from build123d import *

# Parameters (mm, degrees)
SKETCH1_W            = 35
SKETCH1_H            = 35
BOSS_EXTRUDE1_DEPTH  = 3
SKETCH2_R            = 2.5
CUT_EXTRUDE1_DEPTH   = 25.929901725
LPATTERN1_COUNT      = 2
LPATTERN1_PITCH      = 20
LPATTERN1_COUNT_DIR2 = 2
LPATTERN1_PITCH_DIR2 = 20
SKETCH9_R            = 5
SKETCH10_W           = 35
SKETCH10_H           = 35
BOSS_EXTRUDE2_DEPTH  = 3
SKETCH11_R           = 2.5
CUT_EXTRUDE2_DEPTH   = 146.693169663
LPATTERN4_COUNT      = 2
LPATTERN4_PITCH      = 20
LPATTERN4_COUNT_DIR2 = 2
LPATTERN4_PITCH_DIR2 = 20
FILLET1_R            = 3
FILLET2_R            = 3


with BuildPart() as part:
    # Sketch1 → Boss-Extrude1 (new body)
    with BuildSketch(Plane(origin=(0, 0, 0), x_dir=(0, 0, -1), z_dir=(1, 0, 0))):
        Rectangle(SKETCH1_W, SKETCH1_H)
    extrude(amount=BOSS_EXTRUDE1_DEPTH)

    # Sketch2 → Cut-Extrude1 (cut, through all)
    with BuildSketch(Plane(origin=(3, 0, 0), x_dir=(0, 0, -1), z_dir=(1, 0, 0))):
        with Locations((10, 10)):
            Circle(SKETCH2_R)
    cut_extrude1 = extrude(amount=-CUT_EXTRUDE1_DEPTH, mode=Mode.SUBTRACT)

    # LPattern1: Cut-Extrude1 2 × 2
    with Locations(*[(0, -j * LPATTERN1_PITCH_DIR2, i * LPATTERN1_PITCH) for i in range(LPATTERN1_COUNT) for j in range(LPATTERN1_COUNT_DIR2) if (i, j) != (0, 0)]):
        add(cut_extrude1, mode=Mode.SUBTRACT)

    # Sweep1: sweep along a path in Sketch8
    with BuildLine(Plane.XY) as sweep1_path:
        Line((3, 0), (50, 0))
        ThreePointArc((50, 0), (67.677670206, 7.32233044), (75.000001, 25.0000005))
        Line((75.000001, 25.0000005), (75.000001, 90))
        ThreePointArc((75.000001, 90), (67.677670383, 107.677669883), (50.0000005, 115.0000005))
        Line((50.0000005, 115.0000005), (25.0000005, 115.0000005))
    # Sketch9 → Sweep1 (sweep)
    with BuildSketch(Plane(origin=(3, 0, 0), x_dir=(0, 0, -1), z_dir=(1, 0, 0))):
        Circle(SKETCH9_R)
    sweep(path=sweep1_path.line)

    # Sketch10 → Boss-Extrude2 (add)
    with BuildSketch(Plane(origin=(25.000002799, 5e-07, 0), x_dir=(0, 0, 1), z_dir=(-0.9999999999999998, -1.9990267318907433e-08, 0))):
        with Locations((0, 114.9999995)):
            Rectangle(SKETCH10_W, SKETCH10_H)
    extrude(amount=BOSS_EXTRUDE2_DEPTH)

    # Sketch11 → Cut-Extrude2 (cut, through all)
    with BuildSketch(Plane(origin=(22.000002799, 4.4e-07, 0), x_dir=(0, 0, 1), z_dir=(-0.9999999999999998, -1.999026737793079e-08, 0))):
        with Locations(Location((9.998977528, 124.998977028, 0), (0, 0, 270))):
            Circle(SKETCH11_R)
    cut_extrude2 = extrude(amount=-CUT_EXTRUDE2_DEPTH, mode=Mode.SUBTRACT)

    # LPattern4: Cut-Extrude2 2 × 2
    with Locations(*[(0, -j * LPATTERN4_PITCH_DIR2, -i * LPATTERN4_PITCH) for i in range(LPATTERN4_COUNT) for j in range(LPATTERN4_COUNT_DIR2) if (i, j) != (0, 0)]):
        add(cut_extrude2, mode=Mode.SUBTRACT)

    # Fillet1
    fillet1_edges = [part.edges().sort_by_distance(p)[0] for p in [
        (25.0000005, 115.0000005, 5),
    ]]
    fillet(fillet1_edges, radius=FILLET1_R)

    # Fillet2
    fillet2_edges = [part.edges().sort_by_distance(p)[0] for p in [
        (3, 0, 5),
    ]]
    fillet(fillet2_edges, radius=FILLET2_R)


solid = part.part
The listing builds one solid part. Answer for the finished solid, in the listing's coordinates (mm). A direction names the side the tool comes from. Round coordinates to 2 decimals unless told otherwise and drop trailing zeros. Order: outer loops, then holes, each group sorted by start corner. A loop starts at its lowest first (then second) coordinate and runs counter-clockwise, first axis right, second up. Notation, with made-up numbers: (63.5, -13) -> (112.5, -13) arc R7 ccw to (112.5, -6) -> close; hole circle Ø5 at (35, 68.5). An arc over 180 degrees is marked (long way). Put each result on its own line as item: value.
Q1. Section B-B, the plane y = 10 is taken. Count the separate pieces of the cut face and the enclosed holes in it, and give its area (3 significant figures).
Results list:
separate pieces: 4
enclosed holes: 0
area: 175 mm^2
Q2. Each of these flat-tipped pins is pushed along its axis until it touches: P1, Ø0.9, axis at x = 2, z = 2.5, coming from the +Y side; P2, Ø3, axis at y = 125, z = -10, coming from the +X side; P3, Ø6.5, axis at y = 105, z = -10, coming from the +X side; P4, Ø12, axis at y = 81, z = 6.5, coming from the +X side. Where does it stop, or does it pass through?
Results list:
P1: y = 17.5
P2: through
P3: x = 25
P4: x = 79.97
Q3. Section C-C, the plane x = 14.5 is taken. Write down the section's boundary in (y, z).
Results list:
outline: circle Ø10 at (0, 0)
Q4. Consider line 1 along Y through (x, z) = (2.1, 10); line 2 along Y through (x, z) = (33, 0.5); line 3 along Y through (x, z) = (22.5, 5.5). Determine where each line is inside the solid, lowest interval first.
Results list:
line 1: -17.5 to -12.5, -7.5 to 7.5, 12.5 to 17.5
line 2: -4.97 to 4.97, 110.03 to 119.97
line 3: 97.5 to 132.5
Q5. Determine the mould class of faces 6 (the flat face through (0, 0, 0)), 7 (the cylindrical face through (23.479, 107.497, -9.891)), 8 (the flat face through (1, -17.5, 0)) for opening direction Y: pulls with the +Y half, pulls with the -Y half, needs draft (parallel to the pull), parting line crosses it, or undercut.
Results list:
face 6: needs draft
face 7: undercut
face 8: pulls with the -Y half
Q6. Section A-A, the plane y = -10 is taken. Write down the section's boundary in (x, z).
Results list:
outline: (0, -17.5) -> (3, -17.5) -> (3, -12.5) -> (0, -12.5) -> close; (0, -7.5) -> (3, -7.5) -> (3, 7.5) -> (0, 7.5) -> close; (0, 12.5) -> (3, 12.5) -> (3, 17.5) -> (0, 17.5) -> close
Q7. Which of the six approach directions +Z, -Z, +X, -X, +Y, -Y give full straight-line access (tool end or side, diameter ignored) to faces 1 (the flat face through (22, 115, 0)), 2 (the cylindrical face through (1.52, 7.56, 10.54)), 3 (the flat face through (24, 97.5, 0)), 4 (the flat face through (1, 0, -17.5)), 5 (the cylindrical face through (28.31, -4.88, 1.08))?
Results list:
face 1: +Z, -Z, -X, +Y
face 2: +X, -X
face 3: +Z, -Z, -X
face 4: -Z, +X, -X, +Y, -Y
face 5: none
